CAD build for the part. Positions are in the model's coordinates, mm. A direction names the side the tool comes from. Round coordinates to 2 decimals unless told otherwise and drop trailing zeros. Loops run counter-clockwise (first coordinate to the right, second up) from the corner with the lowest first, then second, coordinate; pieces in that order, holes last.
```python
from build123d import *

# Parameters (mm, degrees)
ESQUISSE1_R      = 0.75
EXTRUSION1_DEPTH = 1


with BuildPart() as part:
    # Esquisse1 → Extrusion1 (new body)
    with BuildSketch(Plane.XY):
        with BuildLine():
            Line((-7.809424908, 6.552045147), (-7.137842505, 9.711591939))
            ThreePointArc((-7.137842505, 9.711591939), (-7.093293962, 9.816702497), (-7.012703099, 9.897559869))
            ThreePointArc((-7.012703099, 9.897559869), (-5.753680876, 10.647078732), (-4.415601587, 11.244120857))
            ThreePointArc((-4.415601587, 11.244120857), (-4.184471882, 11.23610854), (-4.027719362, 11.066068))
            Line((-4.027719362, 11.066068), (-3.008027786, 8.26448842))
            ThreePointArc((-3.008027786, 8.26448842), (-3.015921319, 8.039750525), (-3.177778678, 7.883636386))
            ThreePointArc((-3.177778678, 7.883636386), (0, -8.5), (3.177778678, 7.883636386))
            ThreePointArc((3.177778678, 7.883636386), (3.015921319, 8.039750525), (3.008027786, 8.26448842))
            Line((3.008027786, 8.26448842), (4.027719362, 11.066068))
            ThreePointArc((4.027719362, 11.066068), (4.184471882, 11.23610854), (4.415601587, 11.244120857))
            ThreePointArc((4.415601587, 11.244120857), (5.753680876, 10.647078732), (7.012703099, 9.897559869))
            ThreePointArc((7.012703099, 9.897559869), (7.093293962, 9.816702497), (7.137842505, 9.711591939))
            Line((7.137842505, 9.711591939), (7.809424908, 6.552045147))
            ThreePointArc((7.809424908, 6.552045147), (7.834486225, 6.480364242), (7.876742606, 6.417272087))
            ThreePointArc((7.876742606, 6.417272087), (0, -10.9), (-7.876742606, 6.417272087))
            ThreePointArc((-7.876742606, 6.417272087), (-7.834486225, 6.480364242), (-7.809424908, 6.552045147))
        make_face()
        with Locations((-5.5, 9)):
            Circle(ESQUISSE1_R, mode=Mode.SUBTRACT)
        with Locations(Location((5.5, 9, 0), (0, 0, 180))):
            Circle(ESQUISSE1_R, mode=Mode.SUBTRACT)
    extrude(amount=EXTRUSION1_DEPTH)


solid = part.part
```
Item 1: Probe line 1 (X direction, y = -0.25, z = 0.8); line 2 (Y direction, x = 5.5, z = 0.3); line 3 (X direction, y = -5.75, z = 0.55). List the from-to ranges inside material, lowest first.
Answers follow:
line 1: x = -10.45 to -8.5, 8.5 to 10.45
line 2: y = -9.34 to -6.48, 6.48 to 8.25, 9.75 to 10.77
line 3: x = -9.01 to -6.26, 6.26 to 9.01
Item 2: 3-axis set-ups, long thin cutter, end or side, ignore diameter. For faces 4 (the flat face through (8, -4, 0)), 5 (the flat face through (-3.525, 9.685, 0.493)): which of +Z, -Z, +X, -X, +Y, -Y reach the whole face in a straight line?
Answers follow:
face 4: -Z, +X, -X, +Y, -Y
face 5: +Z, -Z, +Y
Item 3: Cut at D-D, the plane y = 9. Give the cut face in (x, z), plus the area to 3 significant figures.
Answers follow:
outline: (-7.29, 0) - (-6.25, 0) - (-6.25, 1) - (-7.29, 1) - close; (-4.75, 0) - (-3.28, 0) - (-3.28, 1) - (-4.75, 1) - close; (3.28, 0) - (4.75, 0) - (4.75, 1) - (3.28, 1) - close; (6.25, 0) - (7.29, 0) - (7.29, 1) - (6.25, 1) - close
area: 5.03 mm2
Item 4: Two-plate mould, pull along X, no slides. Class faces 1 (the flat face through (3.511, 9.646, 0.493)), 2 (the flat face through (-7.48, 8.11, 0.49)), 3 (the flat face through (8, -4, 1)): released by +X, released by -X, zero draft, split by the parting line, or undercut.
Answers follow:
face 1: undercut
face 2: released by -X
face 3: zero draft
Item 5: Cut at C-C, the plane x = 6.5. Give the cut face in (y, z), plus the area to 3 significant figures.
Answers follow:
outline: (-8.63, 0) - (-5.48, 0) - (-5.48, 1) - (-8.63, 1) - close; (5.48, 0) - (10.23, 0) - (10.23, 1) - (5.48, 1) - close
area: 7.91 mm2
Item 6: Cut at A-A, the plane z = 0.75. Give the cut face in (x, y), plus the area to 3 significant figures.
Answers follow:
outline: (-7.88, 6.42) arc R10.45 ccw (long way) to (7.88, 6.42) arc R0.3 cw to (7.81, 6.55) - (7.14, 9.71) arc R0.3 ccw to (7.01, 9.9) arc R12.5 ccw to (4.42, 11.24) arc R0.3 ccw to (4.03, 11.07) - (3.01, 8.26) arc R0.3 ccw to (3.18, 7.88) arc R8.5 cw (long way) to (-3.18, 7.88) arc R0.3 ccw to (-3.01, 8.26) - (-4.03, 11.07) arc R0.3 ccw to (-4.42, 11.24) arc R12.5 ccw to (-7.01, 9.9) arc R0.3 ccw to (-7.14, 9.71) - (-7.81, 6.55) arc R0.3 cw to start; hole circle Ø1.5 at (-5.5, 9); hole circle Ø1.5 at (5.5, 9)
area: 120 mm2
Item 7: Cut at B-B, the plane y = -6. Give the cut face in (x, z), plus the area to 3 significant figures.
Answers follow:
outline: (-8.85, 0) - (-6.02, 0) - (-6.02, 1) - (-8.85, 1) - close; (6.02, 0) - (8.85, 0) - (8.85, 1) - (6.02, 1) - close
area: 5.67 mm2
